Geometry check sheet. Reference: the model listing, model coordinates, mm. Face numbers are marked on the shaded views. A direction names the side the tool comes from. Give positions to 0.01 mm unless a question says otherwise; leave off trailing zeros. Loops run counter-clockwise (first coordinate to the right, second up) from the corner with the lowest first, then second, coordinate; pieces in that order, holes last. Notation, with made-up numbers: (37, 40) -> (41, 40) arc R4 ccw to (41, 45) -> close; hole circle Ø6 at (65, 39.25). An arc over 180 degrees is marked (long way). One line per question, with ' | ' between items.
from build123d import *

# Parameters (mm, degrees)
F0_W     = 120
F0_H     = 80
F0_R     = 5
F1_DEPTH = 10
F2_W     = 120
F2_H     = 10
F3_DEPTH = 45
F4_R     = 5
F5_DEPTH = 25
F6_W     = 10
F6_H     = 54.9613343179
F7_DEPTH = 45
F9_DEPTH = 25


# Not quite as in the source:
# - a feature names something its author has since deleted; it is built from what else it names


with BuildPart() as f1:
    # F0 (on Front) → F1 (new body)
    with BuildSketch(Plane.XZ):
        Rectangle(F0_W, F0_H)
        with Locations((-40, 20)):
            Circle(F0_R, mode=Mode.SUBTRACT)
        with Locations((40, 20.0739782304)):
            Circle(F0_R, mode=Mode.SUBTRACT)
    extrude(amount=F1_DEPTH)

    # F2 (on face) → F3 (join)
    with BuildSketch(Plane.XZ.offset(10)):
        with Locations((0, -20)):
            Rectangle(F2_W, F2_H)
    extrude(amount=F3_DEPTH)

    # F4 (on face) → F5 (cut)
    with BuildSketch(Plane.XY.offset(-15)):
        with Locations((-39.2463095486, -32.116651535)):
            Circle(F4_R)
        with Locations((38.7271312058, -32.4570691816)):
            Circle(F4_R)
    extrude(amount=-F5_DEPTH, mode=Mode.SUBTRACT)

    # F6 (on face) → F7 (join)
    with BuildSketch(Plane.XZ.offset(10)):
        with Locations((0.0515476614, 12.480667159)):
            Rectangle(F6_W, F6_H)
    extrude(amount=F7_DEPTH)

    # F8 (on face) → F9 (cut)
    with BuildSketch(Plane(origin=(-4.9484523386, 0, 0), x_dir=(0, -1, 0), z_dir=(-1, 0, 0))):
        Polygon((55, 39.9613343179), (10, 39.9613343179), (55, -15), align=None)
    extrude(amount=-F9_DEPTH, mode=Mode.SUBTRACT)


solid = f1.part
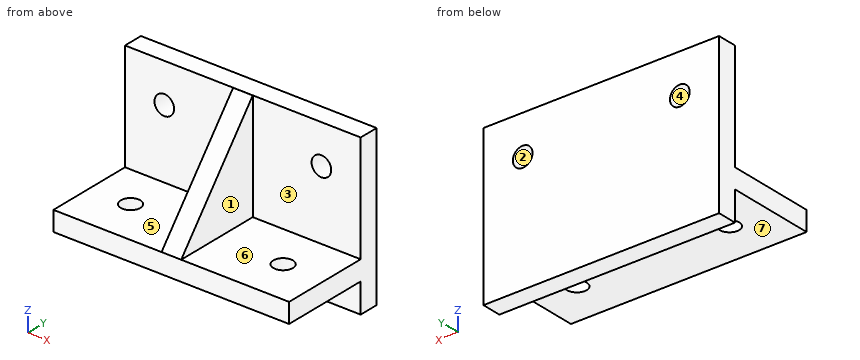
Item 1: Set-up check for the marked faces 4, 5, 6 and 7: record each of +Z, -Z, +X, -X, +Y, -Y from which the full face is reachable in a straight line by a thin tool's end or side.
Result:
face 4: +Y, -Y | face 5: +Z, -X, -Y | face 6: +Z, +X, -Y | face 7: -Z, +X, -X, -Y
Item 2: Sectioned sample at A-A (z = 21.5). Record the cut outline in (x, y), plus the area to 3 significant figures.
Result:
outline: (-60, -10) -> (-44.77, -10) -> (-44.77, 0) -> (-60, 0) -> close; (-35.23, -10) -> (-4.95, -10) -> (-4.95, -25.12) -> (5.05, -25.12) -> (5.05, -10) -> (35.21, -10) -> (35.21, 0) -> (-35.23, 0) -> close; (44.79, -10) -> (60, -10) -> (60, 0) -> (44.79, 0) -> close | area: 1,160 mm2
Item 3: Scan lines: probe 1 along Z at (x, y) = (-40, -3.5); probe 2 along Z at (x, y) = (44, -46); probe 3 along Y at (x, z) = (38, -8). Record each from-to range of solid material in increasing order.
Result:
probe 1: -40 to 15, 25 to 40 | probe 2: -25 to -15 | probe 3: -10 to 0
Item 4: Sectioned sample at C-C (y = -15). Record the cut outline in (x, z).
Result:
outline: (-60, -25) -> (60, -25) -> (60, -15) -> (5.05, -15) -> (5.05, 33.85) -> (-4.95, 33.85) -> (-4.95, -15) -> (-60, -15) -> close
Item 5: Depth check by flat-ended pin: pin 1 Ø6 at (y, z) = (-19, 9.5) entering from -X; pin 2 Ø2 at (x, y) = (-24, -39) entering from -Z; pin 3 Ø22.5 at (x, y) = (-30.5, -21.5) entering from +Z; pin 4 Ø6 at (x, z) = (40, 20.07) entering from +Y. Enter the tip coordinate at first touch or a pass-through.
Result:
pin 1: x = -4.95 | pin 2: z = -25 | pin 3: z = -15 | pin 4: through
Item 6: Sectioned sample at B-B (x = -38). Record the cut outline in (y, z), plus the area to 3 significant figures.
Result:
outline: (-55, -25) -> (-36.96, -25) -> (-36.96, -15) -> (-55, -15) -> close; (-27.27, -25) -> (-10, -25) -> (-10, -40) -> (0, -40) -> (0, 15.42) -> (-10, 15.42) -> (-10, -15) -> (-27.27, -15) -> close; (-10, 24.58) -> (0, 24.58) -> (0, 40) -> (-10, 40) -> close | area: 1,060 mm2
Item 7: Release check for a two-part mould opening along X. For the marked faces 1, 2 and 3 record: pulls with the +X half, pulls with the -X half, needs draft (parallel to the pull), parting line crosses it, or undercut.
Result:
face 1: pulls with the +X half | face 2: undercut | face 3: needs draft
Item 8: Sectioned sample at D-D (x = 11). Record the cut outline in (y, z).
Result:
outline: (-55, -25) -> (-10, -25) -> (-10, -40) -> (0, -40) -> (0, 40) -> (-10, 40) -> (-10, -15) -> (-55, -15) -> close
